Source: three-view drawing plus pictorial views. Frame: mm from the lowest corner of the part. Give positions to 0.01 mm unless a question says otherwise; leave off trailing zeros. Order: outer loops, then holes, each group sorted by start corner. A loop starts at its lowest first (then second) coordinate and runs counter-clockwise, first axis right, second up. Notation, with made-up numbers: (-13.75, 84.5) -> (7.25, 84.5) arc R29 ccw to (7.25, 108.5) -> close; hole circle Ø7 at (-1, 34.5). An arc over 180 degrees is marked (long way). Use a Markdown table: item, result. Add a question column.
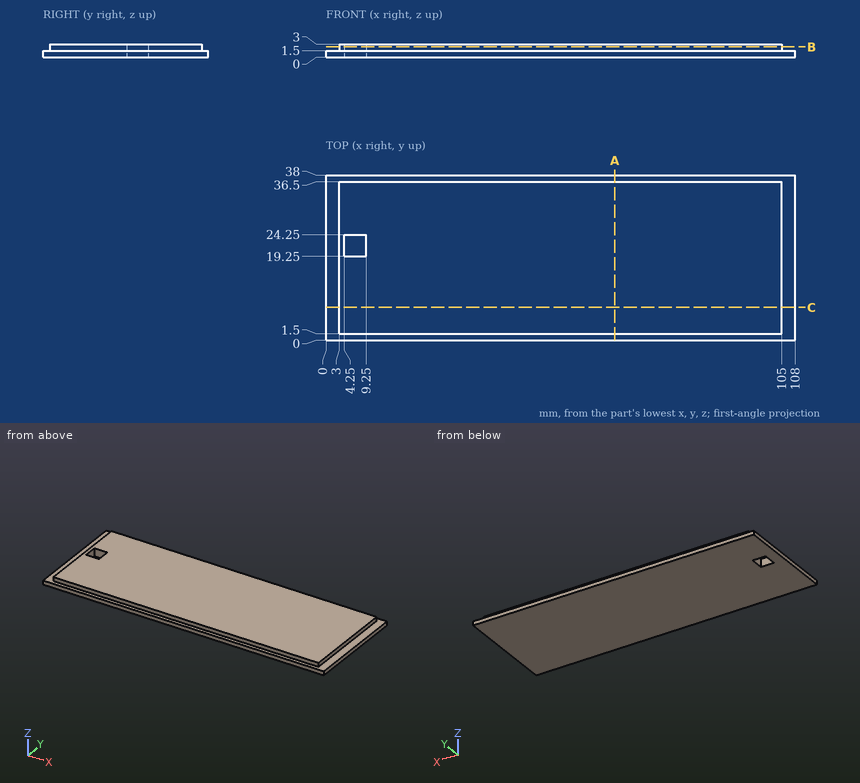
Q1. Section query B-B (z = 2.35). Return loops of the section in (x, y), plus the area to 4 significant figures.
Q2. First-contact query: pin 1 (0.8 mm diameter, centred on x = 30, z = 2.5, fed in from -Y); pin 2 (0.8 mm diameter, centred on x = 61, z = 2, fed in from +Y); pin 3 (0.8 mm diameter, centred on y = 24.5, z = 2.5, fed in from +X). Flat tips, straight axial feed; report the tip coordinate or a pass-through.
Q3. Ray query, line 1 (Y direction, x = 7, z = 0.1); line 2 (Y direction, x = 7, z = 2); line 3 (Y direction, x = 96, z = 1.6). Return the intervals inside material, ascending.
Q4. Section query C-C (y = 7.5). Return loops of the section in (x, z), plus the area to 3 significant figures.
Q5. Section query A-A (x = 66.5). Return loops of the section in (y, z), plus the area to 4 significant figures.
Solution:
| question | item | result |
|---|---|---|
| 1 | outline | (3, 1.5) -> (105, 1.5) -> (105, 36.5) -> (3, 36.5) -> close; hole (4.25, 19.25) -> (9.25, 19.25) -> (9.25, 24.25) -> (4.25, 24.25) -> close |
| 1 | area | 3,545 mm² |
| 2 | pin 1 | stops at y = 1.5 |
| 2 | pin 2 | stops at y = 36.5 |
| 2 | pin 3 | stops at x = 105 |
| 3 | line 1 | y = 0 to 19.25, 24.25 to 38 |
| 3 | line 2 | y = 1.5 to 19.25, 24.25 to 36.5 |
| 3 | line 3 | y = 1.5 to 36.5 |
| 4 | outline | (0, 0) -> (108, 0) -> (108, 1.5) -> (105, 1.5) -> (105, 3) -> (3, 3) -> (3, 1.5) -> (0, 1.5) -> close |
| 4 | area | 315 mm² |
| 5 | outline | (0, 0) -> (38, 0) -> (38, 1.5) -> (36.5, 1.5) -> (36.5, 3) -> (1.5, 3) -> (1.5, 1.5) -> (0, 1.5) -> close |
| 5 | area | 109.5 mm² |
